```python
from build123d import *

# Parameters (mm, degrees)
SKETCH1_W           = 12.446
SKETCH1_H           = 33.02
BOSS_EXTRUDE1_DEPTH = 30.48
SKETCH3_R           = 6.223
BOSS_EXTRUDE2_DEPTH = 3.048
SKETCH4_R           = 3.175
BOSS_EXTRUDE3_DEPTH = 3.81
SKETCH5_R           = 5.715
SKETCH5_R_2         = 3.175
BOSS_EXTRUDE5_DEPTH = 3.048


with BuildPart() as part:
    # Sketch1 → Boss-Extrude1 (new body)
    with BuildSketch(Plane.XY):
        with Locations((6.223, 16.51)):
            Rectangle(SKETCH1_W, SKETCH1_H)
    extrude(amount=BOSS_EXTRUDE1_DEPTH)

    # Sketch3 → Boss-Extrude2 (add)
    with BuildSketch(Plane(origin=(0, 33.02, 0), x_dir=(1, 0, 0), z_dir=(0, 1, 0))):
        with Locations(Location((6.223, -6.223, 0), (0, 0, 90))):
            Circle(SKETCH3_R)
    extrude(amount=BOSS_EXTRUDE2_DEPTH)

    # Sketch4 → Boss-Extrude3 (add)
    with BuildSketch(Plane(origin=(0, 36.068, 0), x_dir=(1, 0, 0), z_dir=(0, 1, 0))):
        with Locations(Location((6.223, -6.223, 0), (0, 0, 90))):
            Circle(SKETCH4_R)
    extrude(amount=BOSS_EXTRUDE3_DEPTH)

    # Sketch5 → Boss-Extrude5 (add)
    # profile 1 of 3: a face of its own
    with BuildSketch(Plane(origin=(0, 36.068, 0), x_dir=(1, 0, 0), z_dir=(0, 1, 0))):
        with Locations((6.223, -6.223)):
            Circle(SKETCH5_R)
        with Locations(Location((6.223, -6.223, 0), (0, 0, 90))):
            Circle(SKETCH5_R_2, mode=Mode.SUBTRACT)
    # profile 2 of 3: a face of its own
    with BuildSketch(Plane(origin=(0, 36.068, 0), x_dir=(1, 0, 0), z_dir=(0, 1, 0))):
        with BuildLine():
            ThreePointArc((0.923781736, -9.485516634), (1.129757079, -2.647443323), (7.491130735, -0.130580658))
            Line((7.491130735, -0.130580658), (-10.085283199, 12.208407524))
            Line((-10.085283199, 12.208407524), (-16.652632198, 2.853471548))
            Line((-16.652632198, 2.853471548), (0.923781736, -9.485516634))
        make_face()
    # profile 3 of 3: a face of its own
    with BuildSketch(Plane(origin=(0, 36.068, 0), x_dir=(1, 0, 0), z_dir=(0, 1, 0))):
        with BuildLine():
            ThreePointArc((2.9393255, -10.900467988), (1.545532012, -2.9393255), (9.5066745, -1.545532012))
            Line((9.5066745, -1.545532012), (7.491130735, -0.130580658))
            ThreePointArc((7.491130735, -0.130580658), (1.129757079, -2.647443323), (0.923781736, -9.485516634))
            Line((0.923781736, -9.485516634), (2.9393255, -10.900467988))
        make_face()
    extrude(amount=BOSS_EXTRUDE5_DEPTH)


solid = part.part
```
Geometry check sheet. Reference: the model listing, model coordinates, mm. A direction names the side the tool comes from. Coordinates: 2 decimals unless noted, no trailing zeros. Loops run counter-clockwise (first coordinate to the right, second up) from the corner with the lowest first, then second, coordinate; pieces in that order, holes last.
Item 1: Release check for a two-part mould opening along Y. For faces 1 (the face through (-13.32, 37.57, -7.6)), 2 (the face through (1, 33.02, 1)), 3 (the face through (-3, 39.116, 0)) record: released by +Y, released by -Y, zero draft, split by the parting line, or undercut.
Item 2: Go/stop test with flat-tipped pins: pin 1 Ø11 at (x, z) = (1, -6) entering from -Y; pin 2 Ø12 at (x, z) = (-1.5, -0.5) entering from +Y; pin 3 Ø4 at (x, z) = (5, 19) entering from +Y; pin 4 Ø12 at (x, z) = (-8, 11) entering from -Y. Record where each tip stops, or that it passes through.
Item 3: Sectioned sample at D-D, the plane z = 16. Record the boundary of the cut face in (x, y), then the cut area to 3 significant figures.
Item 4: Sectioned sample at A-A, the plane z = 7.5. Record the boundary of the cut face in (x, y), then the cut area to 3 significant figures.
Item 5: Sectioned sample at C-C, the plane y = 7.5. Record the boundary of the cut face in (x, z).
Item 6: Access from +Z, -Z, +X, -X, +Y, -Y to the whole of each face (thin tool, end or side, straight path). Record for faces 4 (the face through (4.35, 34.52, 0.29)), 5 (the face through (10.827, 37.571, 9.609)), 6 (the face through (6, 17, 0)), 7 (the face through (6, 17, 30.48)), 8 (the face through (0, 16, 15)).
Item 7: Sectioned sample at B-B, the plane x = 4. Record the boundary of the cut face in (y, z).
Item 8: Thickness scan on line 1 (Y direction, x = -8.75, z = -8.5); line 2 (X direction, y = 4, z = 12); line 3 (Z direction, x = 9, y = 14). Record the ranges inside material, lowest first.
Check result:
1. face 1: zero draft
1. face 2: undercut
1. face 3: released by +Y
2. pin 1: stops at y = 36.07
2. pin 2: stops at y = 39.12
2. pin 3: stops at y = 33.02
2. pin 4: passes through
3. outline: (0, 0) - (12.45, 0) - (12.45, 33.02) - (0, 33.02) - close
3. area: 411 mm2
4. outline: (-1.9, 36.07) - (0.13, 36.07) - (0.13, 33.02) - (0, 33.02) - (0, 0) - (12.45, 0) - (12.45, 33.02) - (12.31, 33.02) - (12.31, 36.07) - (11.79, 36.07) - (11.79, 39.12) - (9.13, 39.12) - (9.13, 39.88) - (3.32, 39.88) - (3.32, 39.12) - (-1.9, 39.12) - close
4. area: 494 mm2
5. outline: (0, 0) - (12.45, 0) - (12.45, 30.48) - (0, 30.48) - close
6. face 4: none
6. face 5: +Y
6. face 6: -Z, +X, -X, -Y
6. face 7: +Z, +X, -X, +Y, -Y
6. face 8: +Z, -Z, -X, -Y
7. outline: (0, 0) - (33.02, 0) - (33.02, 0.41) - (36.07, 0.41) - (36.07, -2.32) - (39.12, -2.32) - (39.12, 3.96) - (39.88, 3.96) - (39.88, 8.49) - (39.12, 8.49) - (39.12, 11.49) - (36.07, 11.49) - (36.07, 12.04) - (33.02, 12.04) - (33.02, 30.48) - (0, 30.48) - close
8. line 1: y = 36.07 to 39.12
8. line 2: x = 0 to 12.45
8. line 3: z = 0 to 30.48
